Can you work these out from the drawing? Everything is in mm from the part's minimum corner. Round coordinates to 2 decimals unless told otherwise and drop trailing zeros. Write each loop counter-clockwise with the first axis right and the second up, starting at its lowest first coordinate (ties: lowest second). Pieces come first, ordered by that corner, then holes. Notation, with made-up numbers: M 69.25,79.5 L 95.25,79.5 A8 cw 95.25,93.5 Z; hole C 18.25,-39.75 d9. An arc over 180 degrees is marked long. Use one line per item in the form item = value. Start each with the question number.
Q1. I'm going to push flat-ended pins straight in: pin 1 Ø3 at (y, z) = (21, 3.5) entering from +X; pin 2 Ø1 at (y, z) = (39, 0.5) entering from +X; pin 3 Ø3 at (x, z) = (2.5, 2) entering from +Y. Where does each tip first touch, or does it pass through?
Q2. I want a section at B-B on y = 85. List the corners of the cut face in (x, z) for me, and give its area (3 significant figures).
Q3. I want a section at C-C on x = 82. List the corners of the cut face in (y, z) for me.
Q4. I need wall thicknesses on line 1 along Y through (x, z) = (88, 5) (1 decimal); line 2 along Y through (x, z) = (24.5, 2.25); line 3 along X through (y, z) = (39.5, 4.5). Which ranges of each line are inside material? Lowest first, please. Write a range as from..to.
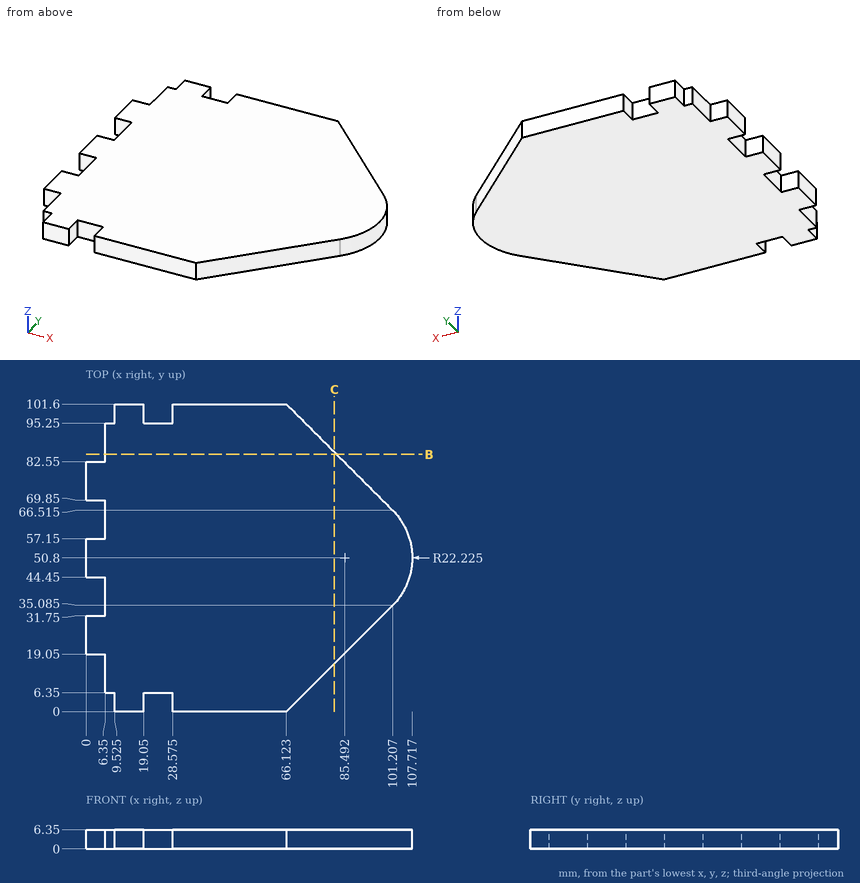
Reported:
q1.pin_1 = 88.62
q1.pin_2 = 104.63
q1.pin_3 = 82.55
q2.outline = M 6.35,0 L 82.72,0 L 82.72,6.35 L 6.35,6.35 Z
q2.area = 485 mm^2
q3.outline = M 15.88,0 L 85.72,0 L 85.72,6.35 L 15.88,6.35 Z
q4.line_1 = 21.9..79.7
q4.line_2 = 6.35..95.25
q4.line_3 = 6.35..104.63
